from build123d import *

# Parameters (mm, degrees)
SKETCH1_W           = 25.4
SKETCH1_H           = 50.8
SKETCH1_W_2         = 20.32
SKETCH1_H_2         = 45.72
EXTRUDE_THIN1_DEPTH = 282.575
SKETCH2_R           = 2.4765
CUT_EXTRUDE1_DEPTH  = 51.8


with BuildPart() as part:
    # Sketch1 → Extrude-Thin1 (new body, symmetric)
    with BuildSketch(Plane(origin=(0, 0, 0), x_dir=(0, 0, -1), z_dir=(1, 0, 0))):
        Rectangle(SKETCH1_W, SKETCH1_H)
        Rectangle(SKETCH1_W_2, SKETCH1_H_2, mode=Mode.SUBTRACT)
    extrude(amount=EXTRUDE_THIN1_DEPTH, both=True)

    # Sketch2 → Cut-Extrude1 (cut, through all)
    with BuildSketch(Plane(origin=(0, 25.4, 0), x_dir=(1, 0, 0), z_dir=(0, 1, 0))):
        with Locations((-269.875, 0)):
            Circle(SKETCH2_R)
        with Locations((-244.475, 0)):
            Circle(SKETCH2_R)
        with Locations((269.875, 0)):
            Circle(SKETCH2_R)
        with Locations((244.475, 0)):
            Circle(SKETCH2_R)
    extrude(amount=-CUT_EXTRUDE1_DEPTH, mode=Mode.SUBTRACT)


solid = part.part
The listing builds one solid part. Answer for the finished solid, in the listing's coordinates (mm). A direction names the side the tool comes from. Round coordinates to 2 decimals unless told otherwise and drop trailing zeros. Loops run counter-clockwise (first coordinate to the right, second up) from the corner with the lowest first, then second, coordinate; pieces in that order, holes last. Notation, with made-up numbers: M -26,55.25 L 12,55.25 A26 cw 12,84.25 Z; hole C 88.25,69 d5. An arc over 180 degrees is marked long. Write each question's results on one line, items separated by ' | '. Start each with the question number.
1) Determine the mould class of faces 1 (the flat face through (-282.575, 2, 10.4)), 2 (the flat face through (4, 0, -10.16)), 3 (the flat face through (4, 25.4, 0)) for opening direction Y: pulls with the +Y half, pulls with the -Y half, needs draft (parallel to the pull), parting line crosses it, or undercut.
2) Find section B-B on x = -191. Write down the section's boundary in (y, z).
3) Which of the six approach directions +Z, -Z, +X, -X, +Y, -Y give full straight-line access (tool end or side, diameter ignored) to faces 4 (the flat face through (4, 0, 10.16)), 5 (the flat face through (4, 0, -12.7))?
4) This flat-tipped pin is pushed along its axis until it touches: pin 1 (3 mm diameter, centred on x = -269.875, z = 0, fed in from -Y). Where does it stop, or does it pass through?
5) Find section A-A on y = 14. Write down the section's boundary in (x, z) (3 decimals).
6) Straight lines are drawn through the part: probe 1 along X at (y, z) = (24.65, 0) (1 decimal); probe 2 along Z at (x, y) = (-53.5, -0.5); probe 3 along Y at (x, z) = (213, 9). For each, find the intervals that lie inside material, in ascending order.
Final values:
1) face 1: needs draft | face 2: undercut | face 3: pulls with the +Y half
2) outline: M -25.4,-12.7 L 25.4,-12.7 L 25.4,12.7 L -25.4,12.7 Z; hole M -22.86,-10.16 L 22.86,-10.16 L 22.86,10.16 L -22.86,10.16 Z
3) face 4: +X, -X | face 5: -Z, +X, -X, +Y, -Y
4) pin 1: through
5) outline: M -282.575,-12.7 L 282.575,-12.7 L 282.575,-10.16 L -282.575,-10.16 Z; M -282.575,10.16 L 282.575,10.16 L 282.575,12.7 L -282.575,12.7 Z
6) probe 1: -282.6 to -272.4, -267.4 to -247, -242 to 242, 247 to 267.4, 272.4 to 282.6 | probe 2: -12.7 to -10.16, 10.16 to 12.7 | probe 3: -25.4 to -22.86, 22.86 to 25.4
